Print and shaded views of the part. All mm, measured from the part's lowest x, y and z. A direction names the side the tool comes from. Round coordinates to 2 decimals unless told otherwise and drop trailing zeros. Write each loop counter-clockwise with the first axis right and the second up, starting at its lowest first coordinate (ties: lowest second). Pieces come first, ordered by that corner, then holes. Notation, with made-up numbers: M -14.5,86.25 L 13.5,86.25 A22 ccw 13.5,115.25 Z; hole C 13.5,42 d5. An arc over 180 degrees is marked long. Write item = value, one per line.
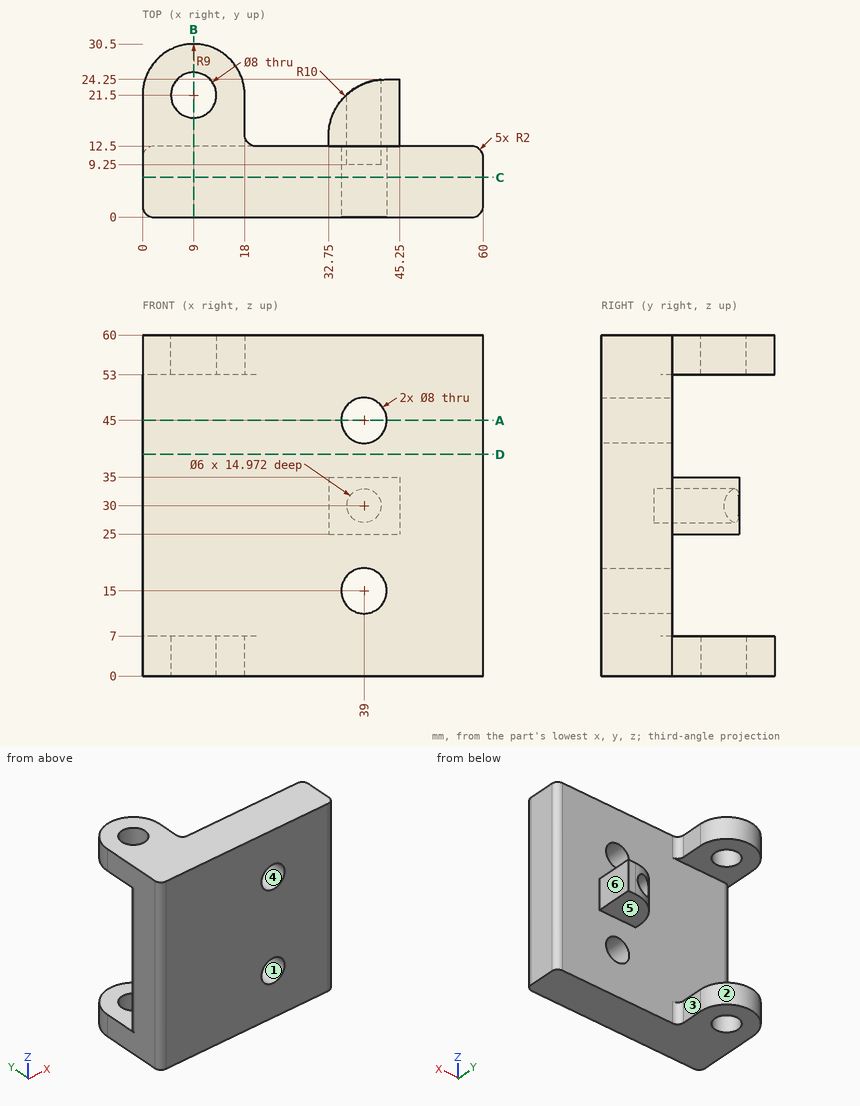
1. Tool access for the marked faces 4, 5 and 6: list every direction of +Z, -Z, +X, -X, +Y, -Y with a clear straight run to the whole face (end or side of a thin tool).
Responses:
face_4 = +Y, -Y
face_5 = -Z, +X, -X, +Y
face_6 = +Z, -Z, +X, +Y
2. Band-saw the part on A-A (z = 45). List the corners of the cut face in (x, y), plus the area to 3 significant figures.
Responses:
outline = M 0,2 A2 ccw 2,0 L 35,0 L 35,12.5 L 2,12.5 A2 ccw 0,10.5 Z; M 43,0 L 58,0 A2 ccw 60,2 L 60,10.5 A2 ccw 58,12.5 L 43,12.5 Z
area = 647 mm²
3. Probe probe 1 along Z at (x, y) = (39, 9); probe 2 along X at (y, z) = (7.5, 15); probe 3 along Y at (x, z) = (16, 42.5). List the from-to ranges inside material, lowest first.
Responses:
probe_1 = 0 to 11, 19 to 41, 49 to 60
probe_2 = 0 to 35, 43 to 60
probe_3 = 0 to 12.5
4. Band-saw the part on B-B (x = 9). List the corners of the cut face in (y, z), plus the area to 3 significant figures.
Responses:
outline = M 0,0 L 17.5,0 L 17.5,7 L 12.5,7 L 12.5,53 L 17.5,53 L 17.5,60 L 0,60 Z; M 25.5,0 L 30.5,0 L 30.5,7 L 25.5,7 Z; M 25.5,53 L 30.5,53 L 30.5,60 L 25.5,60 Z
area = 890 mm²
5. Band-saw the part on D-D (z = 39). List the corners of the cut face in (x, y), plus the area to 3 significant figures.
Responses:
outline = M 0,2 A2 ccw 2,0 L 58,0 A2 ccw 60,2 L 60,10.5 A2 ccw 58,12.5 L 2,12.5 A2 ccw 0,10.5 Z
area = 747 mm²
6. Band-saw the part on C-C (y = 7). List the corners of the cut face in (x, z).
Responses:
outline = M 0,0 L 60,0 L 60,60 L 0,60 Z; hole C 39,15 d8; hole C 39,45 d8
7. Mould opens along X. For the marked faces 1, 2 and 3 say: pulls with the +X half, pulls with the -X half, needs draft (parallel to the pull), parting line crosses it, or undercut.
Responses:
face_1 = undercut
face_2 = parting line crosses it
face_3 = pulls with the +X half
8. Flat gauge pins, fed straight in: pin 1 (5.5 mm diameter, centred on y = 18.5, z = 55.5, fed in from +X); pin 2 (10 mm diameter, centred on y = 23, z = 32.5, fed in from +X); pin 3 (5 mm diameter, centred on x = 45.5, y = 18, fed in from -Z). Where does each tip first touch, or does it go through?
Responses:
pin_1 = 18
pin_2 = 45.25
pin_3 = 25
